from build123d import *

# Parameters (mm, degrees)
CROQUIS1_R              = 20
SALIENTE_EXTRUIR1_DEPTH = 8
CROQUIS2_R              = 5
CORTAR_EXTRUIR1_DEPTH   = 3
REDONDEO1_R             = 2


with BuildPart() as part:
    # Croquis1 → Saliente-Extruir1 (new body)
    with BuildSketch(Plane(origin=(0, 0, 0), x_dir=(1, 0, 0), z_dir=(0, 1, 0))):
        with Locations(Location((0, 0, 0), (0, 0, 270))):
            Circle(CROQUIS1_R)
    extrude(amount=SALIENTE_EXTRUIR1_DEPTH)

    # Croquis2 → Cortar-Extruir1 (cut)
    with BuildSketch(Plane(origin=(0, 8, 0), x_dir=(1, 0, 0), z_dir=(0, 1, 0))):
        with Locations(Location((0, 10, 0), (0, 0, 270))):
            Circle(CROQUIS2_R)
    extrude(amount=-CORTAR_EXTRUIR1_DEPTH, mode=Mode.SUBTRACT)

    # Redondeo1
    redondeo1_edges = [part.edges().sort_by_distance(p)[0] for p in [
        (0, 8, -15),
    ]]
    fillet(redondeo1_edges, radius=REDONDEO1_R)


solid = part.part
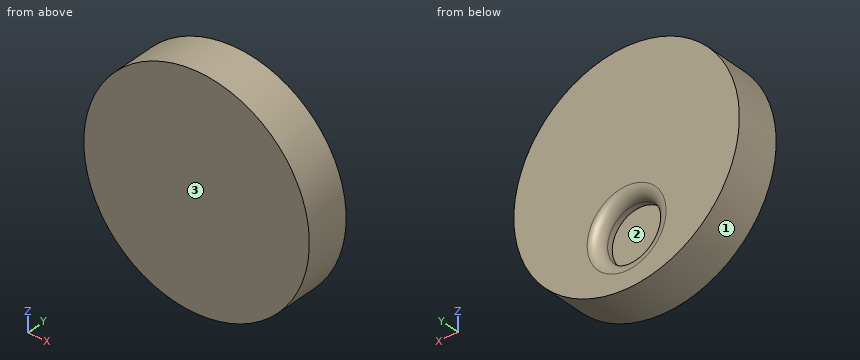
Geometry: final body of the model. Coordinates: model frame, mm. Face numbers are marked on the shaded views. Round coordinates to 2 decimals unless told otherwise and drop trailing zeros. Order: outer loops, then holes, each group sorted by start corner. A loop starts at its lowest first (then second) coordinate and runs counter-clockwise, first axis right, second up.
Q1. Material intervals for probe 1 along X at (y, z) = (5.75, -10); probe 2 along Z at (x, y) = (-0.5, 6.25); probe 3 along Z at (x, y) = (3.5, 7), sorted ascending.
Result sheet:
probe 1: x = -17.32 to -5, 5 to 17.32
probe 2: z = -19.99 to -14.99, -5.01 to 19.99
probe 3: z = -19.69 to -13.94, -6.06 to 19.69
Q2. Mould query, pull axis X, two halves, no side actions, for the marked faces 1, 2 and 3. Classes: released by +X, released by -X, zero draft, split by the parting line, or undercut.
Result sheet:
face 1: split by the parting line
face 2: undercut
face 3: zero draft
Q3. Section C-C, the plane y = 3.25. Output: boundary loops of the cut face in (x, z), and give its area (3 significant figures).
Result sheet:
outline: circle Ø40 at (0, 0)
area: 1,260 mm2
Q4. Section D-D, the plane x = -9. Output: boundary loops of the cut face in (y, z).
Result sheet:
outline: (0, -17.86) - (8, -17.86) - (8, 17.86) - (0, 17.86) - close
Q5. Section A-A, the plane x = 0. Output: boundary loops of the cut face in (y, z), and give its area (3 significant figures).
Result sheet:
outline: (0, -20) - (8, -20) - (8, -17) arc R2 ccw to (6, -15) - (5, -15) - (5, -5) - (6, -5) arc R2 ccw to (8, -3) - (8, 20) - (0, 20) - close
area: 288 mm2
Q6. Section B-B, the plane z = -10. Output: boundary loops of the cut face in (x, y).
Result sheet:
outline: (-17.32, 0) - (17.32, 0) - (17.32, 8) - (7, 8) arc R2 ccw to (5, 6) - (5, 5) - (-5, 5) - (-5, 6) arc R2 ccw to (-7, 8) - (-17.32, 8) - close
Q7. Pin query (flat end, axial travel): pin 1 (2 mm diameter, centred on x = -3, y = 6.5, fed in from -Z); pin 2 (13 mm diameter, centred on x = 0, z = -10, fed in from +Y); pin 3 (4 mm diameter, centred on y = 7, z = -6.5, fed in from +X). Return the tip coordinate at first contact, or that it passes through.
Result sheet:
pin 1: stops at z = -19.9
pin 2: stops at y = 7.94
pin 3: stops at x = 19.49
